from build123d import *

# Parameters (mm, degrees)
SKETCH008_W     = 53.333333
SKETCH008_H     = 46
PAD005_DEPTH    = 3
SKETCH010_W     = 45.333333
SKETCH010_H     = 0.7
PAD006_DEPTH    = 2
POCKET005_DEPTH = 3


with BuildPart() as part:
    # Sketch008 → Pad005 (new body)
    with BuildSketch(Plane.XY.offset(15)):
        with Locations((16.333334, 0)):
            Rectangle(SKETCH008_W, SKETCH008_H)
    extrude(amount=PAD005_DEPTH)

    # Sketch010 → Pad006 (join)
    with BuildSketch(Plane(origin=(0, 0, 15), x_dir=(1, 0, 0), z_dir=(0, 0, -1))):
        with Locations((16.333334, 21.5)):
            Rectangle(SKETCH010_W, SKETCH010_H)
    pad006 = extrude(amount=PAD006_DEPTH)

    # Mirrored001: Pad006 across XZ
    add(pad006.mirror(Plane.XZ))

    # Sketch009 (on Face6 of Pad005) → Pocket005 (cut)
    with BuildSketch(Plane.XY.offset(18)):
        with BuildLine():
            ThreePointArc((0, -4.5), (4.5, 0), (0, 4.5))
            Line((0, 4.5), (-10.333333, 4.5))
            Line((-10.333333, 4.5), (-10.333333, -4.5))
            Line((-10.333333, -4.5), (0, -4.5))
        make_face()
    extrude(amount=-POCKET005_DEPTH, mode=Mode.SUBTRACT)


solid = part.part
Part model, mm, in its own coordinate system. A direction names the side the tool comes from. Give positions to 0.01 mm unless a question says otherwise; leave off trailing zeros. Write each loop counter-clockwise with the first axis right and the second up, starting at its lowest first coordinate (ties: lowest second). Pieces come first, ordered by that corner, then holes.
1) Pin check, flat tips, straight feed: pin 1 (1.6 mm diameter, centred on x = 26.5, z = 14, fed in from +Y); pin 2 (0.6 mm diameter, centred on y = 21.5, z = 14, fed in from +X); pin 3 (8 mm diameter, centred on x = 16, y = -8.5, fed in from -Z). Stop position of each tip, or through.
Resolved:
pin 1: stops at y = 21.85
pin 2: stops at x = 39
pin 3: stops at z = 15
2) Which spindle directions (+Z, -Z, +X, -X, +Y, -Y) get a long thin tool onto all of the face, cutting with end or side? Do faces 1 (the face through (16, -21.85, 14)), 2 (the face through (16, 21.85, 14)), 3 (the face through (-5, -4.5, 17)), 4 (the face through (16, -21.15, 14)). Say none if no direction does.
Resolved:
face 1: -Z, +X, -X, -Y
face 2: -Z, +X, -X, +Y
face 3: +Z, -Z, -X
face 4: -Z, +X, -X
3) Cut at B-B on x = 16.5. Write the cut outline in (y, z), then the cut area to 3 significant figures.
Resolved:
outline: (-23, 15) - (-21.85, 15) - (-21.85, 13) - (-21.15, 13) - (-21.15, 15) - (21.15, 15) - (21.15, 13) - (21.85, 13) - (21.85, 15) - (23, 15) - (23, 18) - (-23, 18) - close
area: 141 mm2
4) Two-plate mould, pull along Y, no slides. Class faces 5 (the face through (4.5, -0.1, 16.5)), 6 (the face through (16, 23, 16)), 7 (the face through (16, 0, 18)): released by +Y, released by -Y, zero draft, split by the parting line, or undercut.
Resolved:
face 5: undercut
face 6: released by +Y
face 7: zero draft
5) Cut at C-C on y = 0. Write the cut outline in (x, z).
Resolved:
outline: (4.5, 15) - (43, 15) - (43, 18) - (4.5, 18) - close
6) Cut at A-A on z = 14. Write the cut outline in (x, y).
Resolved:
outline: (-6.33, -21.85) - (39, -21.85) - (39, -21.15) - (-6.33, -21.15) - close; (-6.33, 21.15) - (39, 21.15) - (39, 21.85) - (-6.33, 21.85) - close
7) Cut at D-D on y = 19. Write the cut outline in (x, z), then the cut area to 3 significant figures.
Resolved:
outline: (-10.33, 15) - (43, 15) - (43, 18) - (-10.33, 18) - close
area: 160 mm2
8) Probe L1, parallel to Y at x = 8.5, z = 14.3; L2, parallel to Y at x = 0, z = 15.25; L3, parallel to Z at x = 31.5, y = 7.5. List the from-to ranges inside material, lowest first.
Resolved:
L1: y = -21.85 to -21.15, 21.15 to 21.85
L2: y = -23 to -4.5, 4.5 to 23
L3: z = 15 to 18
